Can you work these out from the model? Positions are in its coordinate system, mm. A direction names the side the tool comes from. Give positions to 0.01 mm unless a question says otherwise; leave off trailing zeros. Loops run counter-clockwise (first coordinate to the right, second up) from the corner with the lowest first, then second, coordinate; pieces in that order, holes last. Notation, with made-up numbers: (-8.75, 64.25) - (6.25, 64.25) arc R20 ccw to (6.25, 102.25) - close; hole circle Ø2 at (50.5, 76). An arc over 180 degrees is marked (long way). Answer as a JSON object with one key per item and string values.
```python
from build123d import *

# Parameters (mm, degrees)
SKETCH4_R               = 14
SKETCH4_R_2             = 1.625
CIRCULAR_FOOT_DEPTH     = 8
FILLET1_R               = 2
CUT_EXTRUDE1_DEPTH      = 2
CUT_EXTRUDE2_DEPTH      = 22.354156673
CUT_EXTRUDE2_DEPTH_BACK = 22.354156673
SKETCH14_W              = 4
SKETCH14_H              = 4
SKETCH16_R              = 2.625
CUT_EXTRUDE3_DEPTH      = 5


with BuildPart() as part:
    # Sketch4 → Circular Foot (new body)
    with BuildSketch(Plane(origin=(0, 0, 0), x_dir=(0, 0, -1), z_dir=(1, 0, 0))):
        Circle(SKETCH4_R)
        with Locations((-7.424621202, -7.424621202)):
            Circle(SKETCH4_R_2, mode=Mode.SUBTRACT)
        with Locations((7.424621202, -7.424621202)):
            Circle(SKETCH4_R_2, mode=Mode.SUBTRACT)
        with Locations((7.424621202, 7.424621202)):
            Circle(SKETCH4_R_2, mode=Mode.SUBTRACT)
        with Locations((-7.424621202, 7.424621202)):
            Circle(SKETCH4_R_2, mode=Mode.SUBTRACT)
    extrude(amount=CIRCULAR_FOOT_DEPTH)

    # Fillet1
    # the kernel refuses this fillet: 2 mm, written as the material it takes off along each edge
    with BuildSketch(Plane(origin=(8, 0, 0), x_dir=(0, 0, -1), z_dir=(0, -1, 0))) as fillet1_piece_1:
        with BuildLine():
            CenterArc((14 - FILLET1_R, -FILLET1_R), FILLET1_R, 0, 90)
            Line((14 - FILLET1_R, 0), (14, 0))
            Line((14, 0), (14, -FILLET1_R))
        make_face()
    revolve(axis=Axis((8, 0, 0), (1, 0, 0)), mode=Mode.SUBTRACT)

    # Sketch7 → Cut-Extrude1 (cut)
    with BuildSketch(Plane.ZY.offset(-8)):
        Polygon((-5.179255605, -5.179255605), (-8.246482052, -4.357394755), (-10.491847649, -6.602760353), (-9.6699868, -9.6699868), (-6.602760353, -10.491847649), (-4.357394755, -8.246482052), align=None)
        Polygon((6.602760353, -10.491847649), (9.6699868, -9.6699868), (10.491847649, -6.602760353), (8.246482052, -4.357394755), (5.179255605, -5.179255605), (4.357394755, -8.246482052), align=None)
        Polygon((6.602760353, 10.491847649), (4.357394755, 8.246482052), (5.179255605, 5.179255605), (8.246482052, 4.357394755), (10.491847649, 6.602760353), (9.6699868, 9.6699868), align=None)
        Polygon((-4.357394755, 8.246482052), (-6.602760353, 10.491847649), (-9.6699868, 9.6699868), (-10.491847649, 6.602760353), (-8.246482052, 4.357394755), (-5.179255605, 5.179255605), align=None)
    extrude(amount=CUT_EXTRUDE1_DEPTH, mode=Mode.SUBTRACT)

    # Sketch14 → Cut-Extrude2 (cut, two sides: drawn at the far end of the back side and taken through both)
    with BuildSketch(Plane.XY.offset(-CUT_EXTRUDE2_DEPTH_BACK)):
        with Locations((2, 0)):
            Rectangle(SKETCH14_W, SKETCH14_H)
    extrude(amount=CUT_EXTRUDE2_DEPTH + CUT_EXTRUDE2_DEPTH_BACK, mode=Mode.SUBTRACT)

    # Sketch16 → Cut-Extrude3 (cut)
    with BuildSketch(Plane(origin=(0, 0, 0), x_dir=(0, 0, -1), z_dir=(1, 0, 0))):
        with Locations(Location((0, 0, 0), (0, 0, 229.632406456))):
            Circle(SKETCH16_R)
    extrude(amount=CUT_EXTRUDE3_DEPTH, mode=Mode.SUBTRACT)


solid = part.part
```
1) Imagine slicing it at D-D on x = 6.75. Write out the boundary of the cut face in (y, z).
Check sheet entries:
{"outline": "circle Ø27.71 at (0, 0); hole (-10.49, -6.6) - (-9.67, -9.67) - (-6.6, -10.49) - (-4.36, -8.25) - (-5.18, -5.18) - (-8.25, -4.36) - close; hole (-10.49, 6.6) - (-8.25, 4.36) - (-5.18, 5.18) - (-4.36, 8.25) - (-6.6, 10.49) - (-9.67, 9.67) - close; hole (4.36, -8.25) - (6.6, -10.49) - (9.67, -9.67) - (10.49, -6.6) - (8.25, -4.36) - (5.18, -5.18) - close; hole (4.36, 8.25) - (5.18, 5.18) - (8.25, 4.36) - (10.49, 6.6) - (9.67, 9.67) - (6.6, 10.49) - close"}
2) Imagine slicing it at C-C on z = 0. Write out the boundary of the cut face in (x, y) (3 decimals), and give its area (3 significant figures).
Check sheet entries:
{"outline": "(0, -14) - (6, -14) arc R2 ccw to (8, -12) - (8, 12) arc R2 ccw to (6, 14) - (0, 14) - (0, 2.625) - (5, 2.625) - (5, -2.625) - (0, -2.625) - close", "area": "196 mm2"}
3) If we mould it in two halves opening along Z, with no side actions, what happens to faces 5 (the flat face through (2, -2, 8)), 6 (the flat face through (7.01, -5.46, -9.35))? For each: released by +Z, released by -Z, zero draft, split by the parting line, or undercut.
Check sheet entries:
{"face 5": "zero draft", "face 6": "undercut"}
4) Imagine slicing it at B-B on y = 0. Write out the boundary of the cut face in (x, z) (3 decimals), and give its area (3 significant figures).
Check sheet entries:
{"outline": "(4, -14) - (6, -14) arc R2 ccw to (8, -12) - (8, 12) arc R2 ccw to (6, 14) - (4, 14) - (4, 2.625) - (5, 2.625) - (5, -2.625) - (4, -2.625) - close", "area": "105 mm2"}
5) I need wall thicknesses on L1, parallel to Y at x = 3.5, z = 0 (3 decimals); L2, parallel to Y at x = 2.5, z = 8.5; L3, parallel to Y at x = 1.75, z = 2. Which ranges of each line are inside material? Lowest first, please.
Check sheet entries:
{"L1": "-14 to -2.625, 2.625 to 14", "L2": "-11.12 to -8.64, -6.21 to -2, 2 to 6.21, 8.64 to 11.12", "L3": "-13.86 to -2, 2 to 13.86"}
6) Which directions (+Z, -Z, +X, -X, +Y, -Y) give clear straight access to the entire face, cutting with the end or side of a thin tool? Please do faces 1 (the flat face through (4, 0, -8)), 2 (the cylindrical face through (2.958, -8.413, -6.135)), 3 (the cylindrical face through (3.02, -2.42, 1.02)), 4 (the flat face through (6, -9, -6)).
Check sheet entries:
{"face 1": "+Z, -Z, -X", "face 2": "+X, -X", "face 3": "-X", "face 4": "+X"}
7) Imagine slicing it at A-A on x = 1.5. Write out the boundary of the cut face in (y, z) (3 decimals).
Check sheet entries:
{"outline": "(-2, -13.856) - (-2, -1.7) arc R2.625 cw to (-2, 1.7) - (-2, 13.856) arc R14 ccw to start; (2, -13.856) arc R14 ccw to (2, 13.856) - (2, 1.7) arc R2.625 cw to (2, -1.7) - close; hole circle Ø3.25 at (-7.425, -7.425); hole circle Ø3.25 at (-7.425, 7.425); hole circle Ø3.25 at (7.425, -7.425); hole circle Ø3.25 at (7.425, 7.425)"}
8) I'm going to push flat-ended pins straight in: P1, Ø3, axis at x = 2, z = 10, coming from the +Y side; P2, Ø1.8, axis at y = 6, z = 6.5, coming from the +X side; P3, Ø3, axis at x = 1, z = 8, coming from the -Y side; P4, Ø2.5, axis at y = 7.42, z = 7.42, coming from the +X side. Where does each tip first touch, or does it pass through?
Check sheet entries:
{"P1": "y = 11.12", "P2": "x = 6", "P3": "y = -12.4", "P4": "through"}
